```python
from build123d import *

# Parameters (mm, degrees)
SKETCH2_R           = 10
BOSS_EXTRUDE1_DEPTH = 25.4
SKETCH3_R           = 3.175
CUT_EXTRUDE1_DEPTH  = 12.7
CHAMFER1_SIZE       = 0.5
SKETCH4_R           = 4
CUT_EXTRUDE2_DEPTH  = 12.7


with BuildPart() as part:
    # Sketch2 → Boss-Extrude1 (new body)
    with BuildSketch(Plane(origin=(0, 0, 0), x_dir=(1, 0, 0), z_dir=(0, 1, 0))):
        with Locations(Location((0, 0, 0), (0, 0, 270))):
            Circle(SKETCH2_R)
    extrude(amount=BOSS_EXTRUDE1_DEPTH)

    # Sketch3 → Cut-Extrude1 (cut)
    with BuildSketch(Plane(origin=(0, 25.4, 0), x_dir=(1, 0, 0), z_dir=(0, 1, 0))):
        with Locations(Location((0, 0, 0), (0, 0, 270))):
            Circle(SKETCH3_R)
    extrude(amount=-CUT_EXTRUDE1_DEPTH, mode=Mode.SUBTRACT)

    # Chamfer1
    chamfer1_edges = [part.edges().sort_by_distance(p)[0] for p in [
        (0, 0, -10),
        (0, 25.4, -10),
        (0, 25.4, -3.175),
    ]]
    chamfer(chamfer1_edges, length=CHAMFER1_SIZE)

    # Sketch4 → Cut-Extrude2 (cut)
    with BuildSketch(Plane.XZ):
        with Locations(Location((0, 0, 0), (0, 0, 270))):
            Circle(SKETCH4_R)
    extrude(amount=-CUT_EXTRUDE2_DEPTH, mode=Mode.SUBTRACT)


solid = part.part
```
Part model, mm, in its own coordinate system. A direction names the side the tool comes from. Coordinates: 2 decimals unless noted, no trailing zeros. Order: outer loops, then holes, each group sorted by start corner. A loop starts at its lowest first (then second) coordinate and runs counter-clockwise, first axis right, second up. Notation, with made-up numbers: (75, 34) -> (80, 34) arc R22 ccw to (80, 59) -> close; hole circle Ø8 at (89.25, 68). An arc over 180 degrees is marked (long way). Put each result on its own line as item: value. Start each with the question number.
(1) Band-saw the part on A-A (z = 0). Give the cut face in (x, y) (3 decimals).
(2) Probe line 1 along X through (y, z) = (7, 0); line 2 along X through (y, z) = (20, 0) (3 decimals); line 3 along Z through (x, y) = (-0.75, 11.75). List the from-to ranges inside material, lowest first. Write a range as [from, to].
(3) Band-saw the part on C-C (y = 5.5). Give the cut face in (x, z), then the cut area to 3 significant figures.
(4) Pin check, flat tips, straight feed: pin 1 Ø8 at (y, z) = (5.5, -5.5) entering from -X; pin 2 Ø8 at (x, z) = (5.5, 6) entering from -Y; pin 3 Ø1.5 at (x, y) = (-7, 15.5) entering from +Z; pin 4 Ø4 at (y, z) = (21.5, -5.5) entering from -X. Stop position of each tip, or through.
(5) Band-saw the part on B-B (y = 14.5). Give the cut face in (x, z) (3 decimals).
(6) Mould opens along X. For faces 1 (the face through (2, 12.7, 3)), 2 (the face through (-9.76, 12.53, -2.17)), 3 (the face through (-1.93, 18.89, -2.52)), 4 (the face through (-4, 0, 2)) say: pulls with the +X half, pulls with the -X half, needs draft (parallel to the pull), parting line crosses it, or undercut.
(7) Which spindle directions (+Z, -Z, +X, -X, +Y, -Y) get a long thin tool onto all of the face, cutting with end or side? Do faces 5 (the face through (-3.905, 6.261, 0.867)), 6 (the face through (0, 25.4, 4)). Say none if no direction does.
Determined:
1. outline: (-10, 0.5) -> (-9.5, 0) -> (-4, 0) -> (-4, 12.7) -> (-3.175, 12.7) -> (-3.175, 24.9) -> (-3.675, 25.4) -> (-9.5, 25.4) -> (-10, 24.9) -> close; (3.175, 12.7) -> (4, 12.7) -> (4, 0) -> (9.5, 0) -> (10, 0.5) -> (10, 24.9) -> (9.5, 25.4) -> (3.675, 25.4) -> (3.175, 24.9) -> close
2. line 1: x = [-10, -4], [4, 10]
2. line 2: x = [-10, -3.175], [3.175, 10]
2. line 3: z = [-9.97, -3.93], [3.93, 9.97]
3. outline: circle Ø20 at (0, 0); hole circle Ø8 at (0, 0)
3. area: 264 mm²
4. pin 1: stops at x = -9.89
4. pin 2: stops at y = 0
4. pin 3: stops at z = 7.81
4. pin 4: stops at x = -9.37
5. outline: circle Ø20 at (0, 0); hole circle Ø6.35 at (0, 0)
6. face 1: undercut
6. face 2: parting line crosses it
6. face 3: undercut
6. face 4: needs draft
7. face 5: -Y
7. face 6: +Z, -Z, +X, -X, +Y
